The model under review builds one solid part; all positions refer to its coordinate system, in mm. Face numbers are marked on the shaded views. A direction names the side the tool comes from. Round coordinates to 2 decimals unless told otherwise and drop trailing zeros. Order: outer loops, then holes, each group sorted by start corner. A loop starts at its lowest first (then second) coordinate and runs counter-clockwise, first axis right, second up. Notation, with made-up numbers: M 9,22 L 14,22 A25 cw 14,46 Z; hole C 9,75 d3. An arc over 180 degrees is marked long. One line per item, written item: value. Start each with the question number.
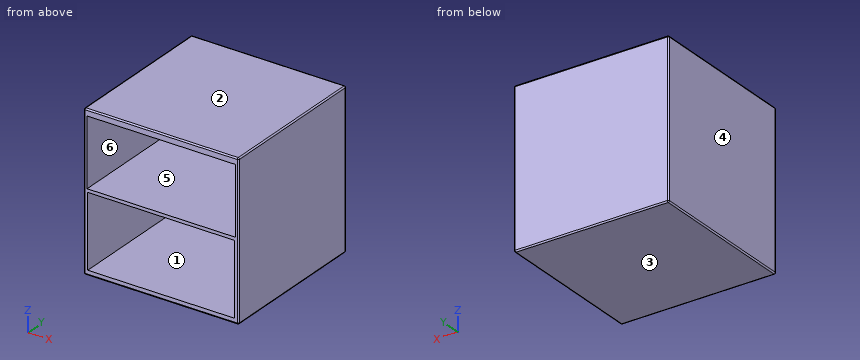
from build123d import *

# Parameters (mm, degrees)
F0_W         = 609.6
F0_H         = 609.6
F1_DEPTH     = 609.6
F3_R         = 5.08
F4_R         = 5.08
F5_T1_DEPTH  = 599.44
F5_T3_DEPTH  = 599.44
F5_T5_DEPTH  = 599.44
F5_S9_W      = 5.08
F5_S9_H      = 5.08
F5_T10_DEPTH = 5.08
F5_S15_W     = 5.08
F5_S15_H     = 5.08
F5_T16_DEPTH = 5.08
F5_S21_W     = 5.08
F5_S21_H     = 5.08
F5_T22_DEPTH = 5.08
F5_S27_W     = 5.08
F5_S27_H     = 5.08
F5_T28_DEPTH = 5.08
F5_T32_ANGLE = 90
F5_T34_ANGLE = 90
F2_W         = 584.2
F2_H         = 266.8860325682
F6_DEPTH     = 596.9
F7_W         = 578.0983269215
F7_H         = 285.4733169079
F8_DEPTH     = 596.9


# Not quite as in the source:
# - a fillet or chamfer that OpenCascade refuses, or shapes differently, is made with other operations: its cross-section is extruded or revolved along the edge and cut away or added


with BuildPart() as f1:
    # F0 (on Front) → F1 (new body)
    with BuildSketch(Plane.XZ):
        Rectangle(F0_W, F0_H)
    extrude(amount=F1_DEPTH)

    # F3
    f3_edges = [f1.edges().sort_by_distance(p)[0] for p in [
        (0, -609.6, 304.8),
    ]]
    fillet(f3_edges, radius=F3_R)

    # F4
    f4_edges = [f1.edges().sort_by_distance(p)[0] for p in [
        (-304.8, -609.6, -2.54),
        (304.8, -609.6, -2.54),
        (0, -609.6, -304.8),
    ]]
    fillet(f4_edges, radius=F4_R)

    # F5: fillet of radius 5.08 on 7 edges, made by hand

    # F5_s2 → F5_t1 (cut)
    with BuildSketch(Plane.XZ.offset(5.08)):
        with BuildLine():
            ThreePointArc((304.8, -299.72), (303.3121024484, -303.3121024484), (299.72, -304.8))
            Line((299.72, -304.8), (304.8, -304.8))
            Line((304.8, -304.8), (304.8, -299.72))
        make_face()
        with BuildLine():
            ThreePointArc((-304.8, -299.72), (-303.3121024484, -303.3121024484), (-299.72, -304.8))
            Line((-299.72, -304.8), (-304.8, -304.8))
            Line((-304.8, -304.8), (-304.8, -299.72))
        make_face()
    extrude(amount=F5_T1_DEPTH, mode=Mode.SUBTRACT)

    # F5_s4 → F5_t3 (cut)
    with BuildSketch(Plane.XY.offset(-299.72)):
        with BuildLine():
            ThreePointArc((299.72, 0), (303.3121024484, -1.4878975516), (304.8, -5.08))
            Line((304.8, -5.08), (304.8, 0))
            Line((304.8, 0), (299.72, 0))
        make_face()
        with BuildLine():
            ThreePointArc((-299.72, 0), (-303.3121024484, -1.4878975516), (-304.8, -5.08))
            Line((-304.8, -5.08), (-304.8, 0))
            Line((-304.8, 0), (-299.72, 0))
        make_face()
    extrude(amount=F5_T3_DEPTH, mode=Mode.SUBTRACT)

    # F5_s6 → F5_t5 (cut)
    with BuildSketch(Plane.YZ.offset(-299.72)):
        with BuildLine():
            ThreePointArc((-5.08, 304.8), (-1.4878975516, 303.3121024484), (0, 299.72))
            Line((0, 299.72), (0, 304.8))
            Line((0, 304.8), (-5.08, 304.8))
        make_face()
        with BuildLine():
            ThreePointArc((0, -299.72), (-1.4878975516, -303.3121024484), (-5.08, -304.8))
            Line((-5.08, -304.8), (0, -304.8))
            Line((0, -304.8), (0, -299.72))
        make_face()
    extrude(amount=F5_T5_DEPTH, mode=Mode.SUBTRACT)


with BuildPart() as f5_tool8:
    # F5_s9 → F5_t10 (new body)
    with BuildSketch(Plane.YZ.offset(-299.72)):
        with Locations((-607.06, -302.26)):
            Rectangle(F5_S9_W, F5_S9_H)
    extrude(amount=-F5_T10_DEPTH)

    # F5_s11 → F5_t12 (revolve, cut)
    with BuildSketch(Plane(origin=(-299.72, -604.52, -299.72), x_dir=(0, 0.7071067812, 0.7071067812), z_dir=(0, -0.7071067812, 0.7071067812))):
        with BuildLine():
            ThreePointArc((0, -5.08), (5.08, 0), (0, 5.08))
            Line((0, 5.08), (0, -5.08))
        make_face()
    revolve(axis=Axis((-299.72, -604.52, -299.72), (-1, 0, 0)), mode=Mode.SUBTRACT)


with BuildPart() as f1_1:
    add(f1.part)

    # F5_t7: cut F5_tool8
    add(f5_tool8.part, mode=Mode.SUBTRACT)


with BuildPart() as f5_tool14:
    # F5_s15 → F5_t16 (new body)
    with BuildSketch(Plane.YZ.offset(299.72)):
        with Locations((-607.06, -302.26)):
            Rectangle(F5_S15_W, F5_S15_H)
    extrude(amount=F5_T16_DEPTH)

    # F5_s17 → F5_t18 (revolve, cut)
    with BuildSketch(Plane(origin=(299.72, -604.52, -299.72), x_dir=(0, 0.7071067812, 0.7071067812), z_dir=(0, 0.7071067812, -0.7071067812))):
        with BuildLine():
            ThreePointArc((0, -5.08), (5.08, 0), (0, 5.08))
            Line((0, 5.08), (0, -5.08))
        make_face()
    revolve(axis=Axis((299.72, -604.52, -299.72), (1, 0, 0)), mode=Mode.SUBTRACT)


with BuildPart() as f1_2:
    add(f1_1.part)

    # F5_t13: cut F5_tool14
    add(f5_tool14.part, mode=Mode.SUBTRACT)


with BuildPart() as f5_tool20:
    # F5_s21 → F5_t22 (new body)
    with BuildSketch(Plane.YZ.offset(299.72)):
        with Locations((-2.54, -302.26)):
            Rectangle(F5_S21_W, F5_S21_H)
    extrude(amount=F5_T22_DEPTH)

    # F5_s23 → F5_t24 (revolve, cut)
    with BuildSketch(Plane(origin=(299.72, -5.08, -299.72), x_dir=(0, -0.7071067812, 0.7071067812), z_dir=(0, 0.7071067812, 0.7071067812))):
        with BuildLine():
            ThreePointArc((0, -5.08), (5.08, 0), (0, 5.08))
            Line((0, 5.08), (0, -5.08))
        make_face()
    revolve(axis=Axis((299.72, -5.08, -299.72), (1, 0, 0)), mode=Mode.SUBTRACT)


with BuildPart() as f1_3:
    add(f1_2.part)

    # F5_t19: cut F5_tool20
    add(f5_tool20.part, mode=Mode.SUBTRACT)


with BuildPart() as f5_tool26:
    # F5_s27 → F5_t28 (new body)
    with BuildSketch(Plane.YZ.offset(-299.72)):
        with Locations((-2.54, -302.26)):
            Rectangle(F5_S27_W, F5_S27_H)
    extrude(amount=-F5_T28_DEPTH)

    # F5_s29 → F5_t30 (revolve, cut)
    with BuildSketch(Plane(origin=(-299.72, -5.08, -299.72), x_dir=(0, -0.7071067812, 0.7071067812), z_dir=(0, -0.7071067812, -0.7071067812))):
        with BuildLine():
            ThreePointArc((0, -5.08), (5.08, 0), (0, 5.08))
            Line((0, 5.08), (0, -5.08))
        make_face()
    revolve(axis=Axis((-299.72, -5.08, -299.72), (-1, 0, 0)), mode=Mode.SUBTRACT)


with BuildPart() as f1_4:
    add(f1_3.part)

    # F5_t25: cut F5_tool26
    add(f5_tool26.part, mode=Mode.SUBTRACT)

    # F5_s31 → F5_t32 (revolve, cut)
    with BuildSketch(Plane.XY.offset(299.72)):
        with BuildLine():
            ThreePointArc((-304.8, -5.08), (-303.3121024484, -1.4878975516), (-299.72, 0))
            Line((-299.72, 0), (-304.8, 0))
            Line((-304.8, 0), (-304.8, -5.08))
        make_face()
    revolve(axis=Axis((-299.72, 0, 299.72), (0, 1, 0)), revolution_arc=F5_T32_ANGLE, mode=Mode.SUBTRACT)

    # F5_s33 → F5_t34 (revolve, cut)
    with BuildSketch(Plane.XY.offset(299.72)):
        with BuildLine():
            ThreePointArc((304.8, -5.08), (303.3121024484, -1.4878975516), (299.72, 0))
            Line((299.72, 0), (304.8, 0))
            Line((304.8, 0), (304.8, -5.08))
        make_face()
    revolve(axis=Axis((299.72, 0, 299.72), (0, -1, 0)), revolution_arc=F5_T34_ANGLE, mode=Mode.SUBTRACT)

    # F2 (on face) → F6 (cut)
    with BuildSketch(Plane.XZ.offset(609.6)):
        with Locations((0, 145.9569837159)):
            Rectangle(F2_W, F2_H)
    extrude(amount=-F6_DEPTH, mode=Mode.SUBTRACT)

    # F7 (on face) → F8 (cut)
    with BuildSketch(Plane.XZ.offset(609.6)):
        with Locations((-0.5959719419, -142.7366584539)):
            Rectangle(F7_W, F7_H)
    extrude(amount=-F8_DEPTH, mode=Mode.SUBTRACT)


solid = f1_4.part
Item 1: The part is to be moulded in two halves that separate along X. For the marked faces 3, 4, 5 and 6, say which applies: pulls with the +X half, pulls with the -X half, needs draft (parallel to the pull), parting line crosses it, or undercut.
Item 2: Clearance check with a flat-ended pin moving along its axis: P1, Ø5, axis at x = -182, z = 53, coming from the -Y side. State where the tip first meets the part, or that it passes through.
Item 3: Consider section D-D, the plane z = -217. Give the boundary of the cut face in (x, y).
Item 4: Consider section B-B, the plane z = 31. Give the boundary of the cut face in (x, y).
Item 5: Machinability: for the marked faces 1 and 2, which of the approach directions +Z, -Z, +X, -X, +Y, -Y give a long, thin tool a straight path to every point of the face, cutting with its end or side? Answer none if there is none.
Item 6: Wall thickness on L1, parallel to Z at x = -38, y = -220; L2, parallel to X at y = -500.5, z = 118.5; L3, parallel to X at y = -448, z = -39: over which ranges is each line inside the solid? List them lowest first.
Item 7: Consider section A-A, the plane y = -499. Give the boundary of the cut face in (x, z), then the cut area to 3 significant figures.
Item 8: Consider section C-C, the plane x = -43. Give the boundary of the cut face in (y, z).
Computed:
1. face 3: needs draft
1. face 4: pulls with the -X half
1. face 5: undercut
1. face 6: undercut
2. P1: stops at y = -12.7
3. outline: M -304.8,-604.52 A5.08 ccw -299.72,-609.6 L -289.65,-609.6 L -289.65,-12.7 L 288.45,-12.7 L 288.45,-609.6 L 299.72,-609.6 A5.08 ccw 304.8,-604.52 L 304.8,-5.08 A5.08 ccw 299.72,0 L -299.72,0 A5.08 ccw -304.8,-5.08 Z
4. outline: M -304.8,-604.52 A5.08 ccw -299.72,-609.6 L -292.1,-609.6 L -292.1,-12.7 L 292.1,-12.7 L 292.1,-609.6 L 299.72,-609.6 A5.08 ccw 304.8,-604.52 L 304.8,-5.08 A5.08 ccw 299.72,0 L -299.72,0 A5.08 ccw -304.8,-5.08 Z
5. face 1: -Y
5. face 2: +Z, +X, -X, +Y, -Y
6. L1: z = -304.8 to -285.47, 0 to 12.51, 279.4 to 304.8
6. L2: x = -304.8 to -292.1, 292.1 to 304.8
6. L3: x = -304.8 to -289.65, 288.45 to 304.8
7. outline: M -304.8,-299.72 A5.08 ccw -299.72,-304.8 L 299.72,-304.8 A5.08 ccw 304.8,-299.72 L 304.8,299.72 A5.08 ccw 299.72,304.8 L -299.72,304.8 A5.08 ccw -304.8,299.72 Z; hole M -292.1,12.51 L 292.1,12.51 L 292.1,279.4 L -292.1,279.4 Z; hole M -289.65,-285.47 L 288.45,-285.47 L 288.45,0 L -289.65,0 Z
7. area: 50,600 mm^2
8. outline: M -609.6,-299.72 A5.08 ccw -604.52,-304.8 L -5.08,-304.8 A5.08 ccw 0,-299.72 L 0,299.72 A5.08 ccw -5.08,304.8 L -604.52,304.8 A5.08 ccw -609.6,299.72 L -609.6,279.4 L -12.7,279.4 L -12.7,12.51 L -609.6,12.51 L -609.6,0 L -12.7,0 L -12.7,-285.47 L -609.6,-285.47 Z
